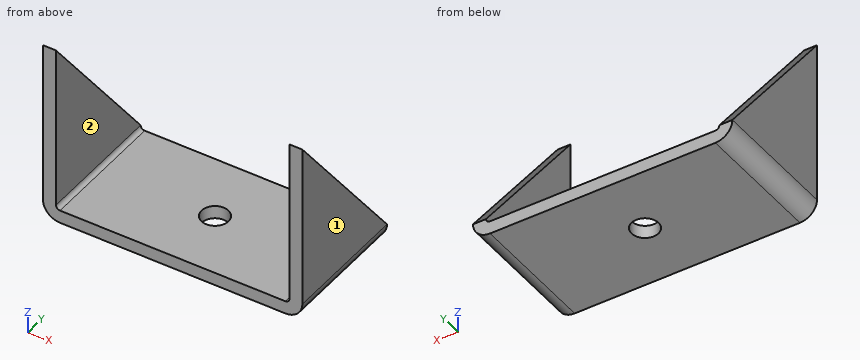
```python
from build123d import *

# Parameters (mm, degrees)
SKETCH2_W                    = 57.15
SKETCH2_H                    = 31.75
BASE_FLANGE1_DEPTH           = 3.175
EDGE_FLANGE1_STRIP_W         = 14.7
EDGE_FLANGE1_STRIP_H         = 3.175
EDGE_FLANGE1_STRIP_CUT_DEPTH = 31.75
EDGE_FLANGE1_DEPTH           = 31.75
CUT_EXTRUDE1_DEPTH           = 3.175
M6_CLEARANCE_HOLE1_D         = 6.6


# Sheet-metal steps are written as plain solids
with BuildPart() as part:
    # Sketch2 → Base-Flange1 (new body)
    with BuildSketch(Plane.XY):
        Rectangle(SKETCH2_W, SKETCH2_H)
    extrude(amount=BASE_FLANGE1_DEPTH)

    # Edge-Flange1 strip (across the edge) → Edge-Flange1 strip cut (cut)
    with BuildSketch(Plane(origin=(28.575, -15.875, 3.175), x_dir=(-1, 0, 0), z_dir=(0, 1, 0))):
        with Locations((-6.35, -1.5875)):
            Rectangle(EDGE_FLANGE1_STRIP_W, EDGE_FLANGE1_STRIP_H)
    edge_flange1_strip_cut = extrude(amount=EDGE_FLANGE1_STRIP_CUT_DEPTH, mode=Mode.SUBTRACT)

    # Edge-Flange1 section (across the edge) → Edge-Flange1 (add)
    with BuildSketch(Plane(origin=(28.575, -15.875, 3.175), x_dir=(-1, 0, 0), z_dir=(0, 1, 0))):
        with BuildLine():
            Line((-3.175, 1), (-3.175, 41.275))
            Line((-3.175, 41.275), (0, 41.275))
            Line((0, 41.275), (0, 1))
            ThreePointArc((0, 1), (0.292893219, 0.292893219), (1, 0))
            Line((1, 0), (1, -3.175))
            ThreePointArc((1, -3.175), (-1.952170811, -1.952170811), (-3.175, 1))
        make_face()
    edge_flange1 = extrude(amount=EDGE_FLANGE1_DEPTH)

    # Sketch10 → Cut-Extrude1 (cut)
    with BuildSketch(Plane(origin=(31.75, 0, 0), x_dir=(0, 0, -1), z_dir=(1, 0, 0))):
        Polygon((-4.175, 15.875), (-44.45, -15.875), (-44.45, 15.875), align=None)
    cut_extrude1 = extrude(amount=-CUT_EXTRUDE1_DEPTH, mode=Mode.SUBTRACT)

    # Mirror1: Edge-Flange1 strip cut, Edge-Flange1, Cut-Extrude1 across plane
    add(edge_flange1_strip_cut.mirror(Plane(origin=(0, 0, 0), x_dir=(0, 0, 1), z_dir=(1, 0, 0))), mode=Mode.SUBTRACT)
    add(edge_flange1.mirror(Plane(origin=(0, 0, 0), x_dir=(0, 0, 1), z_dir=(1, 0, 0))))
    add(cut_extrude1.mirror(Plane(origin=(0, 0, 0), x_dir=(0, 0, 1), z_dir=(1, 0, 0))), mode=Mode.SUBTRACT)

    # M6 Clearance Hole1 (through all)
    with Locations(Plane.XY.offset(3.175)):
        with Locations((0, 0)):
            Hole(M6_CLEARANCE_HOLE1_D / 2)


solid = part.part
```
Build history of the part. All positions in model axes, mm. Face numbers are marked on the shaded views. A direction names the side the tool comes from. Coordinates: 2 decimals unless noted, no trailing zeros. Order: outer loops, then holes, each group sorted by start corner. A loop starts at its lowest first (then second) coordinate and runs counter-clockwise, first axis right, second up. Notation, with made-up numbers: (-14, 78.25) -> (3, 78.25) arc R23 cw to (3, 91.25) -> close; hole circle Ø11 at (20, 45.25). An arc over 180 degrees is marked (long way). Answer in a Markdown table with one row per item. Add a question column.
Q1. Drop a flat-ended pin along its axis: pin 1 (12 mm diameter, centred on x = 14.5, z = 14.5, fed in from +Y). Give the stop position or say it passes through.
Q2. Which spindle directions (+Z, -Z, +X, -X, +Y, -Y) get a long thin tool onto all of the face, cutting with end or side? Do the marked faces 1 and 2. Say none if no direction does.
Q3. Wall check: line 1 along X through (y, z) = (-11.5, 8) (3 decimals); line 2 along Y through (x, z) = (0, 2.45) (3 decimals); line 3 along Z through (x, y) = (-3.5, 13) (3 decimals). Give the ranges that are in metal, low to high. Write a range as [from, to].
Q4. Band-saw the part on C-C, the plane y = -11.5. List the corners of the cut face in (x, z) (3 decimals), then the cut area to 3 significant figures.
Q5. Band-saw the part on A-A, the plane x = 0. List the corners of the cut face in (y, z) (3 decimals).
Q6. Band-saw the part on B-B, the plane z = 18. List the corners of the cut face in (x, y) (3 decimals), then the cut area to 3 significant figures.
Q7. Band-saw the part on D-D, the plane x = -21.5. List the corners of the cut face in (y, z) (3 decimals).
Answers follow:
| question | item | result |
|---|---|---|
| 1 | pin 1 | through |
| 2 | face 1 | +Z, -Z, +X, +Y, -Y |
| 2 | face 2 | +Z, +Y, -Y |
| 3 | line 1 | [-31.75, -28.575], [28.575, 31.75] |
| 3 | line 2 | [-15.875, -3.3], [3.3, 15.875] |
| 3 | line 3 | [0, 3.175] |
| 4 | outline | (-31.75, 4.175) arc R4.175 ccw to (-27.575, 0) -> (27.575, 0) arc R4.175 ccw to (31.75, 4.175) -> (31.75, 38.9) -> (28.575, 38.9) -> (28.575, 4.175) arc R1 cw to (27.575, 3.175) -> (-27.575, 3.175) arc R1 cw to (-28.575, 4.175) -> (-28.575, 38.9) -> (-31.75, 38.9) -> close |
| 4 | area | 421 mm^2 |
| 5 | outline | (-15.875, 0) -> (-3.3, 0) -> (-3.3, 3.175) -> (-15.875, 3.175) -> close; (3.3, 0) -> (15.875, 0) -> (15.875, 3.175) -> (3.3, 3.175) -> close |
| 6 | outline | (-31.75, -15.875) -> (-28.575, -15.875) -> (-28.575, 4.976) -> (-31.75, 4.976) -> close; (28.575, -15.875) -> (31.75, -15.875) -> (31.75, 4.976) -> (28.575, 4.976) -> close |
| 6 | area | 132 mm^2 |
| 7 | outline | (-15.875, 0) -> (15.875, 0) -> (15.875, 3.175) -> (-15.875, 3.175) -> close |
